from build123d import *

# Parameters (mm, degrees)
SKETCH1_W           = 76.08
SKETCH1_H           = 56.08
SKETCH1_W_2         = 71
SKETCH1_H_2         = 51
BOSS_EXTRUDE1_DEPTH = 25.4
SKETCH2_W           = 76.08
SKETCH2_H           = 56.08
BOSS_EXTRUDE2_DEPTH = 2.54
CUT_EXTRUDE1_REACH  = 99.869
CUT_EXTRUDE2_REACH  = 99.869
SKETCH5_R           = 0.75
BOSS_EXTRUDE3_DEPTH = 5
FILLET1_R           = 2.54
CUT_EXTRUDE3_REACH  = 99.869
SKETCH6_W           = 13
SKETCH6_H           = 10
BOSS_EXTRUDE4_DEPTH = 76.08
CHAMFER1_SIZE       = 0.635
SKETCH9_R           = 12.5
CUT_EXTRUDE4_DEPTH  = 101.539100877


with BuildPart() as part:
    # Sketch1 → Boss-Extrude1 (new body)
    with BuildSketch(Plane(origin=(0, 0, 0), x_dir=(1, 0, 0), z_dir=(0, 1, 0))):
        with Locations((38.04, 28.04)):
            Rectangle(SKETCH1_W, SKETCH1_H)
        with Locations((38.04, 28.04)):
            Rectangle(SKETCH1_W_2, SKETCH1_H_2, mode=Mode.SUBTRACT)
    extrude(amount=BOSS_EXTRUDE1_DEPTH)

    # Sketch2 → Boss-Extrude2 (add)
    with BuildSketch(Plane.XZ):
        with Locations((38.04, -28.04)):
            Rectangle(SKETCH2_W, SKETCH2_H)
    extrude(amount=BOSS_EXTRUDE2_DEPTH)

    # Sketch3 → Cut-Extrude1 (cut, up to next)
    with BuildSketch(Plane(origin=(0, 0, -56.08), x_dir=(-1, 0, 0), z_dir=(0, 0, -1)), mode=Mode.PRIVATE) as cut_extrude1_sk1:
        with BuildLine():
            Line((-68.0155, 18.400004), (-68.0155, 25.4))
            Line((-68.0155, 25.4), (-54.6805, 25.4))
            Line((-54.6805, 25.4), (-54.6805, 18.400004))
            ThreePointArc((-54.6805, 18.400004), (-61.348, 11.732504), (-68.0155, 18.400004))
        make_face()
    cut_extrude1_tool1 = extrude(cut_extrude1_sk1.sketch, amount=-CUT_EXTRUDE1_REACH, mode=Mode.PRIVATE) & part.part
    add(cut_extrude1_tool1.solids().sort_by_distance((61.348, 19.19119, -56.08))[0], mode=Mode.SUBTRACT)

    # Cut-Extrude2: up to this face of the body (flat: up to its plane)
    cut_extrude2_end = Plane(part.part.faces().sort_by_distance((73.54, 12.7, -28.04))[0])
    # Sketch4 → Cut-Extrude2 (cut, up to the picked face)
    with BuildSketch(Plane.ZY, mode=Mode.PRIVATE) as cut_extrude2_sk1:
        Polygon((-53.54, 25.4), (-53.54, 24.359997), (-54.54, 24.359997), (-54.54, 22.86), (-1.54, 22.86), (-1.54, 24.359997), (-2.54, 24.359997), (-2.54, 25.4), align=None)
    cut_extrude2_tool1 = split(extrude(cut_extrude2_sk1.sketch, amount=-CUT_EXTRUDE2_REACH, mode=Mode.PRIVATE), bisect_by=cut_extrude2_end, keep=Keep.BOTH, mode=Mode.PRIVATE)
    add(cut_extrude2_tool1.solids().sort_by(Axis((0, 24.11823, -28.04), (1, 0, 0)))[0], mode=Mode.SUBTRACT)

    # Sketch5 → Boss-Extrude3 (add)
    with BuildSketch(Plane(origin=(0, 0, 0), x_dir=(1, 0, 0), z_dir=(0, 1, 0))):
        with Locations(Location((4.893, 51.28999999, 0), (0, 0, 90))):
            Circle(SKETCH5_R)
        with Locations(Location((4.893, 4.79000001, 0), (0, 0, 90))):
            Circle(SKETCH5_R)
        with Locations(Location((71.187, 4.79000001, 0), (0, 0, 90))):
            Circle(SKETCH5_R)
        with Locations(Location((71.187, 51.28999999, 0), (0, 0, 90))):
            Circle(SKETCH5_R)
    extrude(amount=BOSS_EXTRUDE3_DEPTH)

    # Fillet1
    # the kernel refuses this fillet: 2.54 mm, written as the material it adds along each edge
    with BuildSketch(Plane(origin=(4.893, 0, -51.28999999), x_dir=(0, 0, -1), z_dir=(1, 0, 0))) as fillet1_piece_1:
        with BuildLine():
            CenterArc((0.75 + FILLET1_R, FILLET1_R), FILLET1_R, 180, 90)
            Line((0.75, FILLET1_R), (0.75, 0))
            Line((0.75, 0), (0.75 + FILLET1_R, 0))
        make_face()
    revolve(axis=Axis((4.893, 0, -51.28999999), (0, 1, 0)))
    with BuildSketch(Plane(origin=(4.893, 0, -4.79000001), x_dir=(0, 0, -1), z_dir=(1, 0, 0))) as fillet1_piece_2:
        with BuildLine():
            CenterArc((0.75 + FILLET1_R, FILLET1_R), FILLET1_R, 180, 90)
            Line((0.75, FILLET1_R), (0.75, 0))
            Line((0.75, 0), (0.75 + FILLET1_R, 0))
        make_face()
    revolve(axis=Axis((4.893, 0, -4.79000001), (0, 1, 0)))
    with BuildSketch(Plane(origin=(71.187, 0, -4.79000001), x_dir=(0, 0, -1), z_dir=(1, 0, 0))) as fillet1_piece_3:
        with BuildLine():
            CenterArc((0.75 + FILLET1_R, FILLET1_R), FILLET1_R, 180, 90)
            Line((0.75, FILLET1_R), (0.75, 0))
            Line((0.75, 0), (0.75 + FILLET1_R, 0))
        make_face()
    revolve(axis=Axis((71.187, 0, -4.79000001), (0, 1, 0)))
    with BuildSketch(Plane(origin=(71.187, 0, -51.28999999), x_dir=(0, 0, -1), z_dir=(1, 0, 0))) as fillet1_piece_4:
        with BuildLine():
            CenterArc((0.75 + FILLET1_R, FILLET1_R), FILLET1_R, 180, 90)
            Line((0.75, FILLET1_R), (0.75, 0))
            Line((0.75, 0), (0.75 + FILLET1_R, 0))
        make_face()
    revolve(axis=Axis((71.187, 0, -51.28999999), (0, 1, 0)))

    # Sketch6 → Cut-Extrude3 (cut, up to next)
    with BuildSketch(Plane.XY, mode=Mode.PRIVATE) as cut_extrude3_sk1:
        with Locations((20.32, 20.4)):
            Rectangle(SKETCH6_W, SKETCH6_H)
    cut_extrude3_tool1 = extrude(cut_extrude3_sk1.sketch, amount=-CUT_EXTRUDE3_REACH, mode=Mode.PRIVATE) & part.part
    add(cut_extrude3_tool1.solids().sort_by_distance((20.32, 20.4, 0))[0], mode=Mode.SUBTRACT)

    # Sketch7 → Boss-Extrude4 (add)
    with BuildSketch(Plane.ZY):
        Polygon((-56.08, -0.54), (-58.62, -0.54), (-58.62, -2.54), (-60.62, -2.54), (-60.62, 7.46), (-58.62, 7.46), (-58.62, 5.46), (-56.08, 5.46), align=None)
    extrude(amount=-BOSS_EXTRUDE4_DEPTH)

    # Chamfer1
    chamfer1_edges = [part.edges().sort_by_distance(p)[0] for p in [
        (38.04, -2.54, -58.62),
        (38.04, -2.54, -60.62),
        (38.04, 7.46, -60.62),
        (38.04, 7.46, -58.62),
    ]]
    chamfer(chamfer1_edges, length=CHAMFER1_SIZE)

    # Sketch9 → Cut-Extrude4 (cut, through all)
    with BuildSketch(Plane(origin=(0, 0, 0), x_dir=(1, 0, 0), z_dir=(0, 1, 0))):
        with Locations(Location((38.04, 28.04, 0), (0, 0, 270))):
            Circle(SKETCH9_R)
    extrude(amount=-CUT_EXTRUDE4_DEPTH, mode=Mode.SUBTRACT)


solid = part.part
Input: part model. Units: mm. Frame: model coordinates. A direction names the side the tool comes from. Round coordinates to 2 decimals unless told otherwise and drop trailing zeros. Loops run counter-clockwise (first coordinate to the right, second up) from the corner with the lowest first, then second, coordinate; pieces in that order, holes last. Notation, with made-up numbers: M 21,-9.5 L 44,-9.5 A10 ccw 44,-0.5 Z; hole C 27.25,-11 d6. An arc over 180 degrees is marked long. Answer as CSV lines item,"result". Start each with the question number.
(1) Line query: line 1 (Z direction, x = 13.5, y = 8); line 2 (X direction, y = 14, z = -24); line 3 (X direction, y = -0.8, z = -28.04). Output: solid intervals per line, ascending. Write a range as [from, to].
(2) Section A-A, the plane z = -28.04. Output: boundary loops of the cut face in (x, y), plus the area to 3 significant figures.
(3) Section C-C, the plane y = 19.25. Output: boundary loops of the cut face in (x, z).
(4) Reachability of faces 4 (the flat face through (30, 0, -16)), 5 (the flat face through (38, 16, -56.08)), 6 (the cylindrical face through (61.201, 11.734, -54.828)), 7 (the flat face through (20, 15.4, -1)), 8 (the flat face through (38, -0.54, -57)) from +Z, -Z, +X, -X, +Y, -Y: full face, straight path, thin tool, end or side. Return the list, or none.
(5) Section D-D, the plane y = 3.5. Output: boundary loops of the cut face in (x, z), plus the area to 3 significant figures.
(6) First-contact query: pin 1 (0.8 mm diameter, centred on x = 71, z = -5, fed in from +Y); pin 2 (10 mm diameter, centred on y = 11.5, z = -52, fed in from -X); pin 3 (0.7 mm diameter, centred on x = 7, y = 23.5, fed in from -Z); pin 4 (1 mm diameter, centred on x = 30.5, z = -52, fed in from +Y). Flat tips, straight axial feed; report the tip coordinate or a pass-through.
(7) Draft query along X for faces 1 (the flat face through (0, 9, -31)), 2 (the flat face through (54.68, 22, -55)), 3 (the flat face through (27, 25.4, -55)). Return one class per face: released by +X, released by -X, zero draft, split by the parting line, or undercut.
Values found:
1,line 1,"z = [-56.08, -53.54], [-2.54, 0]"
1,line 2,"x = [0, 2.54], [73.54, 76.08]"
1,line 3,"x = [0, 25.54], [50.54, 76.08]"
2,outline,"M 0,-2.54 L 25.54,-2.54 L 25.54,0 L 2.54,0 L 2.54,22.86 L 0,22.86 Z; M 50.54,-2.54 L 76.08,-2.54 L 76.08,25.4 L 73.54,25.4 L 73.54,0 L 50.54,0 Z"
2,area,"252 mm²"
3,outline,"M 0,-56.08 L 54.68,-56.08 L 54.68,-53.54 L 2.54,-53.54 L 2.54,-2.54 L 13.82,-2.54 L 13.82,0 L 0,0 Z; M 26.82,-2.54 L 73.54,-2.54 L 73.54,-53.54 L 68.02,-53.54 L 68.02,-56.08 L 76.08,-56.08 L 76.08,0 L 26.82,0 Z"
4,face 4,"+Y"
4,face 5,"+X, -X, +Y"
4,face 6,"-Z, +Y"
4,face 7,"+Z, +Y"
4,face 8,"+X, -X, -Y"
5,outline,"M 0,-60.62 L 76.08,-60.62 L 76.08,0 L 0,0 Z; C 4.89,-51.29 d1.5; C 4.89,-4.79 d1.5; C 71.19,-51.29 d1.5; C 71.19,-4.79 d1.5; hole M 2.54,-53.54 L 73.54,-53.54 L 73.54,-2.54 L 2.54,-2.54 Z"
5,area,"998 mm²"
6,pin 1,"stops at y = 5"
6,pin 2,"stops at x = 0"
6,pin 3,"stops at z = -56.08"
6,pin 4,"stops at y = 0"
7,face 1,"released by -X"
7,face 2,"undercut"
7,face 3,"zero draft"
